CAD build for the part. Positions are in the model's coordinates, mm. Face numbers are marked on the shaded views. A direction names the side the tool comes from. Give positions to 0.01 mm unless a question says otherwise; leave off trailing zeros. Write each loop counter-clockwise with the first axis right and the second up, starting at its lowest first coordinate (ties: lowest second). Pieces come first, ordered by that corner, then holes. Notation, with made-up numbers: (13.5, 12) - (67.5, 12) arc R20 cw to (67.5, 38) - close; hole circle Ø8 at (14, 35.25). An arc over 180 degrees is marked (long way). Put each result on its own line as item: value. Start each with the question number.
1. Cut at A-A on x = 20.75. List the corners of the cut face in (y, z).
2. Cut at D-D on y = 0. List the corners of the cut face in (x, z), and give its area (3 significant figures).
3. Wall check: line 1 (Y direction, x = 41.5, z = -1.35); line 2 (Y direction, x = 20.75, z = -6.25); line 3 (X direction, y = -2.5, z = -13.5). Give the ranges that are in metal, low to high.
4. Cut at B-B on x = 41.5. List the corners of the cut face in (y, z).
5. Tool access for the marked faces 1, 2 and 3: list every direction of +Z, -Z, +X, -X, +Y, -Y with a clear straight run to the whole face (end or side of a thin tool).
6. Drop flat-ended pins along their axis: pin 1 (7 mm diameter, centred on x = 3, y = -29, fed in from -Z); pin 2 (2 mm diameter, centred on x = 33, z = -9.5, fed in from -Y); pin 3 (1.5 mm diameter, centred on y = -18, z = -6.5, fed in from -X); pin 4 (0.9 mm diameter, centred on x = -20.5, z = -5, fed in from -Y). Give the stop position or say it passes through.
7. Cut at C-C on y = 11. List the corners of the cut face in (x, z), and give its area (3 significant figures).
from build123d import *

# Parameters (mm, degrees)
SKETCH5_R           = 7
SKETCH5_R_2         = 4.7625
SKETCH5_R_3         = 2.1
SKETCH5_R_4         = 4.1
BOSS_EXTRUDE5_DEPTH = 15
CUT_EXTRUDE1_START  = -2
SKETCH1_W           = 29
SKETCH1_H           = 30
SKETCH1_R           = 7
CUT_EXTRUDE1_DEPTH  = 13
CUT_EXTRUDE2_START  = -13
SKETCH5_3_R         = 6.75
SKETCH5_3_R_2       = 4.1
CUT_EXTRUDE2_DEPTH  = 2
FILLET1_R           = 6
FILLET2_R           = 4
FILLET3_R           = 6
FILLET4_R           = 2
BOSS_EXTRUDE6_START = -12.7
SKETCH5_4_R         = 4.7625
BOSS_EXTRUDE6_DEPTH = 2.3


with BuildPart() as part:
    # Sketch5 → Boss-Extrude5 (new body)
    with BuildSketch(Plane.XY):
        with BuildLine():
            Line((58, 17), (-16.5, 17))
            Line((-16.5, 17), (-25.5, -5))
            Line((-25.5, -5), (-25.5, -13))
            Line((-25.5, -13), (-16.5, -13))
            Line((-16.5, -13), (-16.5, -17))
            Line((-16.5, -17), (-6.624344746, -31.585315674))
            ThreePointArc((-6.624344746, -31.585315674), (0.420970348, -35.08891632), (7.059051341, -30.864278705))
            ThreePointArc((7.059051341, -30.864278705), (20.750000185, -22.649146733), (34.440948834, -30.864279032))
            ThreePointArc((34.440948834, -30.864279032), (41.079029838, -35.08891633), (48.124344746, -31.585315674))
            Line((48.124344746, -31.585315674), (58, -17))
            Line((58, -17), (58, -13))
            Line((58, -13), (67, -13))
            Line((67, -13), (67, -5))
            Line((67, -5), (58, 17))
        make_face()
        Circle(SKETCH5_R, mode=Mode.SUBTRACT)
        with Locations((20.75, -14.649146733)):
            Circle(SKETCH5_R_2, mode=Mode.SUBTRACT)
        with Locations((41.5, 0)):
            Circle(SKETCH5_R, mode=Mode.SUBTRACT)
        with Locations((20.75, 11)):
            Circle(SKETCH5_R_3, mode=Mode.SUBTRACT)
        with Locations((-21.5, -9)):
            Circle(SKETCH5_R_3, mode=Mode.SUBTRACT)
        with Locations((63, -9)):
            Circle(SKETCH5_R_3, mode=Mode.SUBTRACT)
        with Locations((41.5, -25.4)):
            Circle(SKETCH5_R_4, mode=Mode.SUBTRACT)
        with Locations((0, -25.4)):
            Circle(SKETCH5_R_4, mode=Mode.SUBTRACT)
    extrude(amount=-BOSS_EXTRUDE5_DEPTH)

    # Sketch1 → Cut-Extrude1 (cut)
    # profile 1 of 2: a face of its own
    with BuildSketch(Plane.XY.offset(CUT_EXTRUDE1_START)):
        Rectangle(SKETCH1_W, SKETCH1_H)
        Circle(SKETCH1_R, mode=Mode.SUBTRACT)
    # profile 2 of 2: a face of its own
    with BuildSketch(Plane.XY.offset(CUT_EXTRUDE1_START)):
        with Locations((41.5, 0)):
            Rectangle(SKETCH1_W, SKETCH1_H)
        with Locations((41.5, 0)):
            Circle(SKETCH1_R, mode=Mode.SUBTRACT)
    extrude(amount=-CUT_EXTRUDE1_DEPTH, mode=Mode.SUBTRACT)

    # Sketch5<3> → Cut-Extrude2 (cut)
    # profile 1 of 2: a face of its own
    with BuildSketch(Plane.XY.offset(CUT_EXTRUDE2_START)):
        with Locations((41.5, -27.1)):
            Circle(SKETCH5_3_R)
        with Locations((41.5, -25.4)):
            Circle(SKETCH5_3_R_2, mode=Mode.SUBTRACT)
    # profile 2 of 2: a face of its own
    with BuildSketch(Plane.XY.offset(CUT_EXTRUDE2_START)):
        with Locations((0, -27.1)):
            Circle(SKETCH5_3_R)
        with Locations((0, -25.4)):
            Circle(SKETCH5_3_R_2, mode=Mode.SUBTRACT)
    extrude(amount=-CUT_EXTRUDE2_DEPTH, mode=Mode.SUBTRACT)

    # Fillet1
    fillet1_edges = [part.edges().sort_by_distance(p)[0] for p in [
        (-14.5, -15, -8.5),
        (14.5, -15, -8.5),
        (14.5, 15, -8.5),
        (-14.5, 15, -8.5),
        (27, -15, -8.5),
        (56, -15, -8.5),
        (56, 15, -8.5),
        (27, 15, -8.5),
    ]]
    fillet(fillet1_edges, radius=FILLET1_R)

    # Fillet2
    fillet2_edges = [part.edges().sort_by_distance(p)[0] for p in [
        (67, -13, -7.5),
        (-25.5, -13, -7.5),
        (-25.5, -5, -7.5),
        (67, -5, -7.5),
    ]]
    fillet(fillet2_edges, radius=FILLET2_R)

    # Fillet3
    fillet3_edges = [part.edges().sort_by_distance(p)[0] for p in [
        (58, -17, -7.5),
        (-16.5, -17, -7.5),
        (-16.5, 17, -7.5),
        (58, 17, -7.5),
    ]]
    fillet(fillet3_edges, radius=FILLET3_R)

    # Fillet4
    fillet4_edges = [part.edges().sort_by_distance(p)[0] for p in [
        (58, -13, -7.5),
        (-16.5, -13, -7.5),
    ]]
    fillet(fillet4_edges, radius=FILLET4_R)

    # Sketch5<4> → Boss-Extrude6 (add)
    with BuildSketch(Plane.XY.offset(BOSS_EXTRUDE6_START)):
        with Locations((20.75, -14.649146733)):
            Circle(SKETCH5_4_R)
    extrude(amount=-BOSS_EXTRUDE6_DEPTH)


solid = part.part
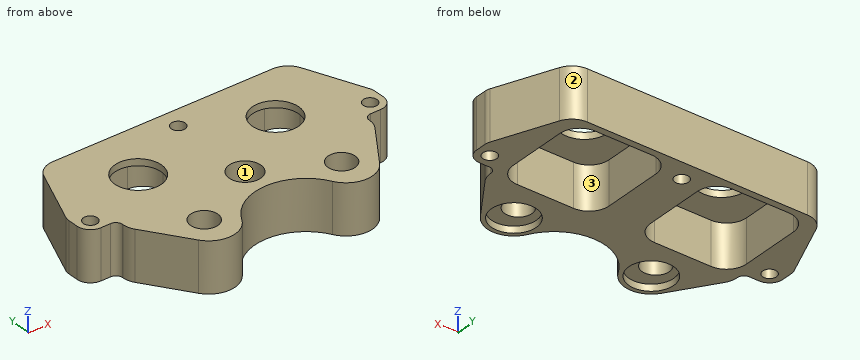
Report:
1. outline: (-22.65, -15) - (8.9, -15) - (8.9, 0) - (-9.89, 0) - (-9.89, -12.7) - (-19.41, -12.7) - (-19.41, 0) - (-22.65, 0) - close; (13.1, -15) - (17, -15) - (17, 0) - (13.1, 0) - close
2. outline: (-23.45, -15) - (-14.5, -15) - (-14.5, -2) - (-7, -2) - (-7, 0) - (-23.45, 0) - close; (7, -2) - (14.5, -2) - (14.5, -15) - (27, -15) - (27, -2) - (34.5, -2) - (34.5, 0) - (7, 0) - close; (48.5, -2) - (56, -2) - (56, -15) - (64.95, -15) - (64.95, 0) - (48.5, 0) - close
2. area: 516 mm²
3. line 1: y = -35.1 to -29.5, -21.3 to -7, 7 to 17
3. line 2: y = -22.65 to -19.41, -9.89 to 8.9, 13.1 to 17
3. line 3: x = -24.48 to -14.5, 14.5 to 27, 56 to 65.98
4. outline: (-35.1, -15) - (-33.85, -15) - (-33.85, -13) - (-29.5, -13) - (-29.5, 0) - (-35.1, 0) - close; (-21.3, -13) - (-20.35, -13) - (-20.35, -15) - (-15, -15) - (-15, -2) - (-7, -2) - (-7, 0) - (-21.3, 0) - close; (7, -2) - (15, -2) - (15, -15) - (17, -15) - (17, 0) - (7, 0) - close
5. face 1: +Z
5. face 2: +Z, -Z, +X, +Y
5. face 3: -Z
6. pin 1: stops at z = -15
6. pin 2: stops at y = -30.09
6. pin 3: stops at x = -16.12
6. pin 4: stops at y = -13
7. outline: (-18.95, -15) - (-14.16, -15) - (-14.16, -2) - (14.16, -2) - (14.16, -15) - (18.65, -15) - (18.65, 0) - (-18.95, 0) - close; (22.85, -15) - (27.34, -15) - (27.34, -2) - (55.66, -2) - (55.66, -15) - (60.45, -15) - (60.45, 0) - (22.85, 0) - close
7. area: 392 mm²
